Here's how the part is built. I have some questions about the finished solid (model axes, mm). Give positions to 0.01 mm unless a question says otherwise; leave off trailing zeros. Loops run counter-clockwise (first coordinate to the right, second up) from the corner with the lowest first, then second, coordinate; pieces in that order, holes last. Notation, with made-up numbers: (54, 60.5) -> (82, 60.5) arc R31 cw to (82, 87.5) -> close; hole circle Ø7 at (73, 60.5). An arc over 180 degrees is marked (long way). Answer in a Markdown table with one row per item. Add a question column.
Item 1: If we section it at B-B (z = 12.5): Give the number of separate pieces and of enclosed holes in the cut face, then the cut area to 3 significant figures.
Item 2: We'd pull the mould along X, two halves only. Please class faces 1 (the face through (0, 2, 20)), 2 (the face through (-26.81, -8.5, 9.86)), 3 (the face through (-16.366, -0.44, 9.86)): released by +X, released by -X, zero draft, split by the parting line, or undercut.
Item 3: If I drill on line 1 (Y direction, x = -12, z = 16); line 2 (Y direction, x = 6, z = 6); line 3 (X direction, y = 7.25, z = 9.75), over which ranges is the centre line in solid material (lowest first)?
Item 4: If we section it at A-A (x = 0): Write out the boundary of the cut face in (y, z), then the cut area to 3 significant figures.
Item 5: For P1, Ø1.4, axis at x = -11.62, y = 0, coming from the -Z side, with a flat end and sliding along its axis, tell me the tip position at first contact or that it passes through.
Item 6: If we section it at D-D (x = 11): Write out the boundary of the cut face in (y, z), then the cut area to 3 significant figures.
```python
from build123d import *

# Parameters (mm, degrees)
SKETCH1_R           = 1.1
SKETCH1_R_2         = 1.15
SKETCH1_R_3         = 1.2
SKETCH1_R_4         = 1.25
SKETCH1_R_5         = 1.3
SKETCH1_R_6         = 1.35
SKETCH1_R_7         = 1.4
SKETCH1_R_8         = 1.45
SKETCH1_R_9         = 1.5
BOSS_EXTRUDE1_DEPTH = 20


with BuildPart() as part:
    # Sketch1 → Boss-Extrude1 (new body)
    with BuildSketch(Plane.XY):
        with BuildLine():
            Line((-23.238249128, -10), (28.238249128, -10))
            Line((28.238249128, -10), (28.238249128, 10))
            Line((28.238249128, 10), (-23.238249128, 10))
            ThreePointArc((-23.238249128, 10), (-26.773783034, 8.535533906), (-28.238249128, 5))
            Line((-28.238249128, 5), (-28.238249128, -5))
            ThreePointArc((-28.238249128, -5), (-26.773783034, -8.535533906), (-23.238249128, -10))
        make_face()
        with Locations((-23.238249128, 0)):
            Circle(SKETCH1_R, mode=Mode.SUBTRACT)
        with Locations((-17.428686846, 0)):
            Circle(SKETCH1_R_2, mode=Mode.SUBTRACT)
        with Locations((-11.619124564, 0)):
            Circle(SKETCH1_R_3, mode=Mode.SUBTRACT)
        with Locations((-5.809562282, 0)):
            Circle(SKETCH1_R_4, mode=Mode.SUBTRACT)
        Circle(SKETCH1_R_5, mode=Mode.SUBTRACT)
        with Locations((5.809562282, 0)):
            Circle(SKETCH1_R_6, mode=Mode.SUBTRACT)
        with Locations((11.619124564, 0)):
            Circle(SKETCH1_R_7, mode=Mode.SUBTRACT)
        with Locations((17.428686846, 0)):
            Circle(SKETCH1_R_8, mode=Mode.SUBTRACT)
        with Locations((23.238249128, 0)):
            Circle(SKETCH1_R_9, mode=Mode.SUBTRACT)
    extrude(amount=BOSS_EXTRUDE1_DEPTH)


solid = part.part
```
Recorded:
| question | item | result |
|---|---|---|
| 1 | separate pieces | 1 |
| 1 | enclosed holes | 9 |
| 1 | area | 1,070 mm^2 |
| 2 | face 1 | zero draft |
| 2 | face 2 | released by -X |
| 2 | face 3 | undercut |
| 3 | line 1 | y = -10 to -1.14, 1.14 to 10 |
| 3 | line 2 | y = -10 to -1.34, 1.34 to 10 |
| 3 | line 3 | x = -27.7 to 28.24 |
| 4 | outline | (-10, 0) -> (-1.3, 0) -> (-1.3, 20) -> (-10, 20) -> close; (1.3, 0) -> (10, 0) -> (10, 20) -> (1.3, 20) -> close |
| 4 | area | 348 mm^2 |
| 5 | P1 | passes through |
| 6 | outline | (-10, 0) -> (-1.26, 0) -> (-1.26, 20) -> (-10, 20) -> close; (1.26, 0) -> (10, 0) -> (10, 20) -> (1.26, 20) -> close |
| 6 | area | 350 mm^2 |
